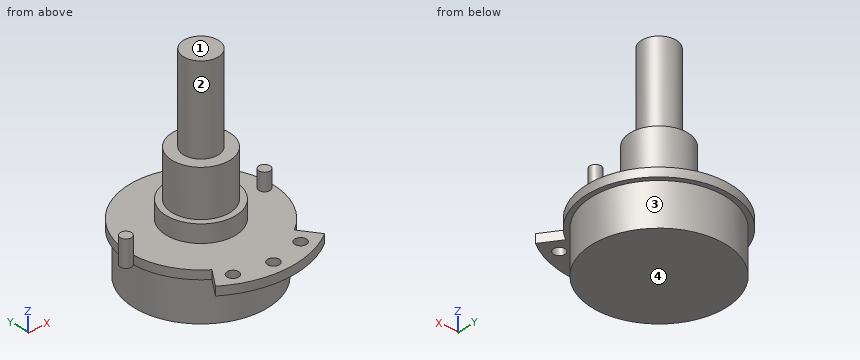
from build123d import *

# Parameters (mm, degrees)
SKETCH1_R      = 11.5
EXTRUDE1_DEPTH = 7.3
EXTRUDE2_DEPTH = 1.5
SKETCH3_R      = 1
EXTRUDE3_DEPTH = 1.5
SKETCH4_R      = 6
EXTRUDE4_DEPTH = 3
SKETCH5_R      = 4.975
EXTRUDE5_DEPTH = 8
SKETCH6_R      = 3
EXTRUDE6_DEPTH = 15
EXTRUDE7_START = -1.5
SKETCH7_R      = 0.95
EXTRUDE7_DEPTH = 4.5


with BuildPart() as part:
    # Sketch1 → Extrude1 (new body)
    with BuildSketch(Plane.XY):
        Circle(SKETCH1_R)
    extrude(amount=EXTRUDE1_DEPTH)

    # Sketch2 → Extrude2 (add)
    with BuildSketch(Plane.XY.offset(7.3)):
        with BuildLine():
            Line((-9.45, -13.342413575), (-7.138073394, -10.078214535))
            ThreePointArc((-7.138073394, -10.078214535), (0, 12.35), (7.138073394, -10.078214535))
            Line((7.138073394, -10.078214535), (9.45, -13.342413575))
            ThreePointArc((9.45, -13.342413575), (0, -16.35), (-9.45, -13.342413575))
        make_face()
    extrude(amount=EXTRUDE2_DEPTH)

    # Sketch3 → Extrude3 (cut)
    with BuildSketch(Plane.XY.offset(8.8)):
        with Locations((0, -14)):
            Circle(SKETCH3_R)
        with Locations((5.860626142, -12.714285714)):
            Circle(SKETCH3_R)
        with Locations((-5.860626142, -12.714285714)):
            Circle(SKETCH3_R)
    extrude(amount=-EXTRUDE3_DEPTH, mode=Mode.SUBTRACT)

    # Sketch4 → Extrude4 (add)
    with BuildSketch(Plane.XY.offset(8.8)):
        Circle(SKETCH4_R)
    extrude(amount=EXTRUDE4_DEPTH)

    # Sketch5 → Extrude5 (add)
    with BuildSketch(Plane.XY.offset(11.8)):
        Circle(SKETCH5_R)
    extrude(amount=EXTRUDE5_DEPTH)

    # Sketch6 → Extrude6 (add)
    with BuildSketch(Plane.XY.offset(19.8)):
        Circle(SKETCH6_R)
    extrude(amount=EXTRUDE6_DEPTH)

    # Sketch7 → Extrude7 (add)
    with BuildSketch(Plane.XY.offset(8.8).offset(EXTRUDE7_START)):
        with Locations((11, 0)):
            Circle(SKETCH7_R)
        with Locations((-13, 0)):
            Circle(SKETCH7_R)
    extrude(amount=EXTRUDE7_DEPTH)


solid = part.part
Check sheet for the modelled part. Datum: model origin and axes. Units: mm. Face numbers are marked on the shaded views. A direction names the side the tool comes from. Round coordinates to 2 decimals unless told otherwise and drop trailing zeros. Order: outer loops, then holes, each group sorted by start corner. A loop starts at its lowest first (then second) coordinate and runs counter-clockwise, first axis right, second up.
(1) Cross-section at C-C, the plane z = 5. Enter the section's corners in (x, y).
(2) Scan lines: probe 1 along Y at (x, z) = (0, 8.2); probe 2 along Z at (x, y) = (-4.5, -7); probe 3 along Z at (x, y) = (0, 5.75). Record each from-to range of solid material in increasing order.
(3) Cross-section at D-D, the plane x = 8.5. Enter the section's corners in (y, z), and give its area (3 significant figures).
(4) Go/stop test with flat-tipped pins: P1, Ø8, axis at x = -10.5, y = 7, coming from the +Z side; P2, Ø3, axis at y = 2.5, z = 21, coming from the -X side; P3, Ø1, axis at x = 1.5, z = 14, coming from the -Y side. Record where each tip stops, or that it passes through.
(5) Cross-section at B-B, the plane y = 0. Enter the section's corners in (x, z) (3 decimals).
(6) Cross-section at A-A, the plane x = 0. Enter the section's corners in (y, z) (3 decimals).
(7) Draft check along X on the marked faces 3 and 4. Enter one of: pulls with the +X half, pulls with the -X half, needs draft (parallel to the pull), parting line crosses it, or undercut.
(8) Access from +Z, -Z, +X, -X, +Y, -Y to the whole of each face (thin tool, end or side, straight path). Record for the marked faces 1 and 2.
Check sheet entries:
1. outline: circle Ø23 at (0, 0)
2. probe 1: y = -16.35 to -15, -13 to 12.35
2. probe 2: z = 0 to 8.8
2. probe 3: z = 0 to 11.8
3. outline: (-13.97, 7.3) - (-12, 7.3) - (-12, 8.8) - (-13.97, 8.8) - close; (-8.96, 7.3) - (-7.75, 7.3) - (-7.75, 0) - (7.75, 0) - (7.75, 7.3) - (8.96, 7.3) - (8.96, 8.8) - (-8.96, 8.8) - close
3. area: 143 mm2
4. P1: stops at z = 8.8
4. P2: stops at x = -4.71
4. P3: stops at y = -4.87
5. outline: (-13.95, 7.3) - (-11.5, 7.3) - (-11.5, 0) - (11.5, 0) - (11.5, 7.3) - (12.35, 7.3) - (12.35, 8.8) - (11.95, 8.8) - (11.95, 11.8) - (10.05, 11.8) - (10.05, 8.8) - (6, 8.8) - (6, 11.8) - (4.975, 11.8) - (4.975, 19.8) - (3, 19.8) - (3, 34.8) - (-3, 34.8) - (-3, 19.8) - (-4.975, 19.8) - (-4.975, 11.8) - (-6, 11.8) - (-6, 8.8) - (-12.05, 8.8) - (-12.05, 11.8) - (-13.95, 11.8) - close
6. outline: (-16.35, 7.3) - (-15, 7.3) - (-15, 8.8) - (-16.35, 8.8) - close; (-13, 7.3) - (-11.5, 7.3) - (-11.5, 0) - (11.5, 0) - (11.5, 7.3) - (12.35, 7.3) - (12.35, 8.8) - (6, 8.8) - (6, 11.8) - (4.975, 11.8) - (4.975, 19.8) - (3, 19.8) - (3, 34.8) - (-3, 34.8) - (-3, 19.8) - (-4.975, 19.8) - (-4.975, 11.8) - (-6, 11.8) - (-6, 8.8) - (-13, 8.8) - close
7. face 3: parting line crosses it
7. face 4: needs draft
8. face 1: +Z, +X, -X, +Y, -Y
8. face 2: +Z
